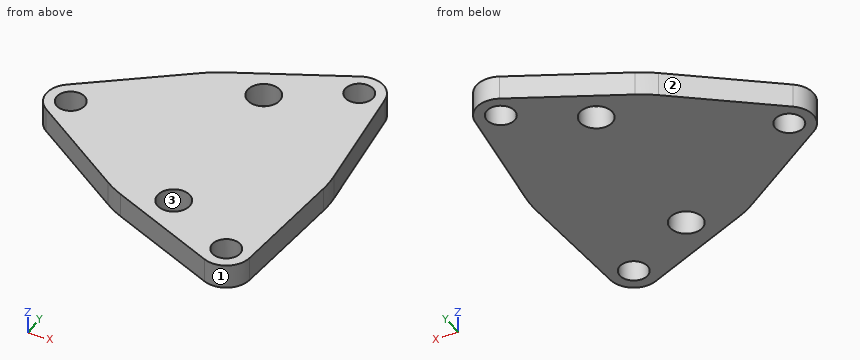
Autodesk Inventor part; units mm, degrees
ref_plane "YZ Plane" through (0, 0, 0) normal (1, 0, 0) x (0, 1, 0)
ref_plane "XZ Plane" through (0, 0, 0) normal (0, 1, 0) x (-1, 0, 0)
ref_plane "XY Plane" through (0, 0, 0) normal (0, 0, 1) x (1, 0, 0)
sketch "Sketch1" plane through (0, 0, 0) normal (0, 0, 1) x (1, 0, 0)
  circle A0 centre (0, 0) radius 14.224
  circle A1 centre (0, 0) radius 19.05 construction
  line L0 (0, 0) -> (-19.05, 0)
  circle A2 centre (-19.05, 0) radius 3.175
  circle A3 centre (0, 11.176) radius 2.1082
  line L1 (0, 0) -> (0, 11.176)
  line L2 (0, 0) -> (0, -11.176)
  circle A4 centre (0, -11.176) radius 2.1082
  line L3 (-20.8915, 2.5864) -> (-8.2499, 11.5871)
  line L4 (-20.8915, -2.5864) -> (-8.2499, -11.5871)
  dimension "d1" = 38.1
  dimension "d0" = 28.448
  dimension "d2" = 6.35
  dimension "d3" = 11.176
  dimension "d4" = 11.176
  dimension "d5" = 4.2164
  dimension "d6" = 4.2164
extrude "Extrusion1" add sketch "Sketch1" along normal blind 3.175 contours A0
extrude "Extrusion2" add sketch "Sketch1" along normal blind 3.175 contours A0 L0 A2 L3 | L4 A2 L0 A0 | A2
hole "Hole1" at (-19.05, 0, 0) direction (0, 0, 1) diameter 3.6576 end through all
pattern_circular "Circular Pattern2" count 3 over 360 about axis through (0, 0, 0) along (0, 0, 1) of "Extrusion2", "Hole1"
properties part number "Mounting Plate"
Here's how the part is built. I have some questions about the finished solid (model axes, mm). Face numbers are marked on the shaded views. Give positions to 0.01 mm unless a question says otherwise; leave off trailing zeros. Order: outer loops, then holes, each group sorted by start corner. A loop starts at its lowest first (then second) coordinate and runs counter-clockwise, first axis right, second up. Notation, with made-up numbers: (14.25, 31) -> (72.25, 31) arc R18 cw to (72.25, 53) -> close; hole circle Ø1 at (38.25, -16). An arc over 180 degrees is marked (long way). Use CSV: the item, a comma, the result in double quotes. Start each with the question number.
Item 1: I'm going to push flat-ended pins straight in: P1, Ø1.5, axis at y = 10.5, z = 0.5, coming from the -X side; P2, Ø1, axis at x = -15, z = 2, coming from the +Y side; P3, Ø1.5, axis at x = -3, z = 1.5, coming from the -Y side. Where does each tip first touch, or does it pass through?
Item 2: If I drill on probe 1 along Y at (x, z) = (9.5, 1.15); probe 2 along Y at (x, z) = (10, 0.4); probe 3 along X at (y, z) = (0, 1.35) (3 decimals), over which ranges is the centre line in solid material (lowest first)? Write a range as [from, to].
Item 3: Suppose I cut it at D-D (z = 1.65). Give the number of separate pieces and of enclosed holes in the cut face, and give its area (3 significant figures).
Item 4: Thinking about a two-plate mould opening in Y: for the marked faces 1, 2 and 3, which applies, pulls with the +Y half, pulls with the -Y half, needs draft (parallel to the pull), parting line crosses it, or undercut?
Item 5: Suppose I cut it at A-A (y = 0). List the corners of the cut face in (x, z) for me (3 decimals), and give its area (3 significant figures).
Item 6: Suppose I cut it at B-B (x = -19.05). List the corners of the cut face in (y, z) for me (3 decimals), and give its area (3 significant figures).
Item 7: Suppose I cut it at C-C (x = 0). List the corners of the cut face in (y, z) for me (3 decimals).
Answer block:
1,P1,"stops at x = -10.83"
1,P2,"stops at y = 7.14"
1,P3,"stops at y = -14.61"
2,probe 1,"y = [-19.67, -18.33], [-14.67, 14.67], [18.33, 19.67]"
2,probe 2,"y = [-19.64, -18.26], [-14.73, 14.73], [18.26, 19.64]"
2,probe 3,"x = [-22.225, -20.879], [-17.221, 14.224]"
3,separate pieces,"1"
3,enclosed holes,"5"
3,area,"837 mm^2"
4,face 1,"pulls with the -Y half"
4,face 2,"pulls with the +Y half"
4,face 3,"undercut"
5,outline,"(-22.225, 0) -> (-20.879, 0) -> (-20.879, 3.175) -> (-22.225, 3.175) -> close; (-17.221, 0) -> (14.224, 0) -> (14.224, 3.175) -> (-17.221, 3.175) -> close"
5,area,"104 mm^2"
6,outline,"(-3.898, 0) -> (-1.829, 0) -> (-1.829, 3.175) -> (-3.898, 3.175) -> close; (1.829, 0) -> (3.898, 0) -> (3.898, 3.175) -> (1.829, 3.175) -> close"
6,area,"13.1 mm^2"
7,outline,"(-15.638, 0) -> (-13.284, 0) -> (-13.284, 3.175) -> (-15.638, 3.175) -> close; (-9.068, 0) -> (9.068, 0) -> (9.068, 3.175) -> (-9.068, 3.175) -> close; (13.284, 0) -> (15.638, 0) -> (15.638, 3.175) -> (13.284, 3.175) -> close"
